Check sheet for the modelled part. Datum: model origin and axes. Units: mm. Coordinates: 2 decimals unless noted, no trailing zeros. Write each loop counter-clockwise with the first axis right and the second up, starting at its lowest first coordinate (ties: lowest second). Pieces come first, ordered by that corner, then holes. Notation, with made-up numbers: (16.25, 78) - (72.25, 78) arc R13 ccw to (72.25, 96) - close; hole circle Ø4 at (22, -33). An arc over 180 degrees is marked (long way). Use one line per item in the form item = value. Start each with the question number.
1. Draft check along Y on faces 1 (the face through (1, 0, 0)), 2 (the face through (3, -5, 11)), 3 (the face through (-2.37, 3.07, 6.9)). Enter one of: +Y half, -Y half, draft (parallel to the pull), parting line (faces both ways), or undercut.
2. Cross-section at A-A on z = 13. Record the boundary of the cut face in (x, y), then the cut area to 3 significant figures.
3. Cross-section at B-B on y = -0.5. Record the boundary of the cut face in (x, z), then the cut area to 3 significant figures.
4. Cross-section at D-D on z = 8.5. Record the boundary of the cut face in (x, y).
5. Cross-section at C-C on x = 2. Record the boundary of the cut face in (y, z), then the cut area to 3 significant figures.
6. Go/stop test with flat-tipped pins: pin 1 Ø3 at (x, y) = (2.5, -1.5) entering from -Z; pin 2 Ø3 at (x, z) = (5, 11.5) entering from +Y. Record where each tip stops, or that it passes through.
7. Scan lines: line 1 along Z through (x, y) = (3, 6.55); line 2 along Y through (x, z) = (3, 10.75); line 3 along Y through (x, z) = (6.35, 8.5). Record each from-to range of solid material in increasing order.
```python
from build123d import *

# Parameters (mm, degrees)
SKETCH_1_W          = 14
SKETCH_1_H          = 14
EXTRUDE_1_DEPTH     = 17
SKETCH_2_R          = 3.1
CUT_EXTRUDE_1_DEPTH = 20.672315573
FILLET_1_R          = 5
CUT_EXTRUDE_2_DEPTH = 17
SKETCH_4_R          = 1.6
CUT_EXTRUDE_3_DEPTH = 17
SKETCH_5_R          = 1.6
CUT_EXTRUDE_4_DEPTH = 17
FILLET_2_R          = 4


with BuildPart() as part:
    # ｽｹｯﾁ1 → ﾎﾞｽ - 押し出し1 (new body)
    with BuildSketch(Plane.XY):
        Rectangle(SKETCH_1_W, SKETCH_1_H)
    extrude(amount=EXTRUDE_1_DEPTH)

    # ｽｹｯﾁ2 → ｶｯﾄ - 押し出し1 (cut, through all)
    with BuildSketch(Plane.XY.offset(17)):
        with Locations((3, 3)):
            Circle(SKETCH_2_R)
    extrude(amount=-CUT_EXTRUDE_1_DEPTH, mode=Mode.SUBTRACT)

    # ﾌｨﾚｯﾄ1
    fillet_1_edges = [part.edges().sort_by_distance(p)[0] for p in [
        (-7, -7, 8.5),
    ]]
    fillet(fillet_1_edges, radius=FILLET_1_R)

    # ｽｹｯﾁ3 → ｶｯﾄ - 押し出し2 (cut)
    with BuildSketch(Plane.XY.offset(17)):
        with BuildLine():
            Line((-7, 7), (-7, -7))
            Line((-7, -7), (7, -7))
            Line((7, -7), (7, -5))
            Line((7, -5), (-2, -5))
            ThreePointArc((-2, -5), (-4.121320344, -4.121320344), (-5, -2))
            Line((-5, -2), (-5, 7))
            Line((-5, 7), (-7, 7))
        make_face()
    extrude(amount=-CUT_EXTRUDE_2_DEPTH, mode=Mode.SUBTRACT)

    # ｽｹｯﾁ4 → ｶｯﾄ - 押し出し3 (cut)
    with BuildSketch(Plane.XZ.offset(5)):
        with Locations(Location((3, 8.5, 0), (0, 0, 270))):
            Circle(SKETCH_4_R)
    extrude(amount=-CUT_EXTRUDE_3_DEPTH, mode=Mode.SUBTRACT)

    # ｽｹｯﾁ5 → ｶｯﾄ - 押し出し4 (cut)
    with BuildSketch(Plane.ZY.offset(5)):
        with Locations((8.5, 3)):
            Circle(SKETCH_5_R)
    extrude(amount=-CUT_EXTRUDE_4_DEPTH, mode=Mode.SUBTRACT)

    # ﾌｨﾚｯﾄ2
    # the kernel refuses this fillet: 4 mm, written as the material it takes off along each edge
    with BuildSketch(Plane(origin=(7, 7, -10), x_dir=(-1, 0, 0), z_dir=(0, 0, 1))) as fillet_2_piece_1:
        with BuildLine():
            CenterArc((FILLET_2_R, FILLET_2_R), FILLET_2_R, 180, 90)
            Line((0, FILLET_2_R), (0, 0))
            Line((0, 0), (FILLET_2_R, 0))
        make_face()
    extrude(amount=37, mode=Mode.SUBTRACT)


solid = part.part
```
Final values:
q1.face_1 = draft
q1.face_2 = -Y half
q1.face_3 = undercut
q2.outline = (-5, -2) arc R3 ccw to (-2, -5) - (7, -5) - (7, 3) arc R4 ccw to (3, 7) - (-5, 7) - close; hole circle Ø6.2 at (3, 3)
q2.area = 108 mm²
q3.outline = (-5, 0) - (7, 0) - (7, 17) - (-5, 17) - close; hole circle Ø3.2 at (3, 8.5)
q3.area = 196 mm²
q4.outline = (-5, -2) arc R3 ccw to (-2, -5) - (1.4, -5) - (1.4, 0.34) arc R3.1 cw to (0.34, 1.4) - (-5, 1.4) - close; (-5, 4.6) - (0.34, 4.6) arc R3.1 cw to (1.4, 5.66) - (1.4, 7) - (-5, 7) - close; (4.6, -5) - (7, -5) - (7, 1.4) - (5.66, 1.4) arc R3.1 cw to (4.6, 0.34) - close; (4.6, 5.66) arc R3.1 cw to (5.66, 4.6) - (6.67, 4.6) arc R4 ccw to (4.6, 6.67) - close
q5.outline = (-5, 0) - (0.07, 0) - (0.07, 7.25) - (-5, 7.25) - close; (-5, 9.75) - (0.07, 9.75) - (0.07, 17) - (-5, 17) - close; (5.93, 0) - (7, 0) - (7, 7.25) - (5.93, 7.25) - close; (5.93, 9.75) - (7, 9.75) - (7, 17) - (5.93, 17) - close
q5.area = 88.9 mm²
q6.pin_1 = 0
q6.pin_2 = 6.97
q7.line_1 = 0 to 6.9, 10.1 to 17
q7.line_2 = -5 to -0.1, 6.1 to 7
q7.line_3 = -5 to 1.4, 4.6 to 5.19
